```python
from build123d import *

# Parameters (mm, degrees)
CROQUIS1_R              = 5
SALIENTE_EXTRUIR1_DEPTH = 12.5
CROQUIS2_R              = 2
SALIENTE_EXTRUIR2_DEPTH = 10
CROQUIS3_R              = 4
SALIENTE_EXTRUIR3_DEPTH = 15
CROQUIS4_W              = 5.65685425
CROQUIS4_H              = 5.65685425
SALIENTE_EXTRUIR4_DEPTH = 10
CROQUIS5_W              = 4
CROQUIS5_H              = 10
CORTAR_EXTRUIR1_DEPTH   = 2
CROQUIS6_R              = 2.5
SALIENTE_EXTRUIR5_DEPTH = 100


with BuildPart() as part:
    # Croquis1 → Saliente-Extruir1 (new, symmetric)
    with BuildSketch(Plane.XY):
        Circle(CROQUIS1_R)
    extrude(amount=SALIENTE_EXTRUIR1_DEPTH, both=True)

    # Croquis2 → Saliente-Extruir2 (add)
    with BuildSketch(Plane(origin=(0, 0, -12.5), x_dir=(-1, 0, 0), z_dir=(0, 0, -1))):
        Circle(CROQUIS2_R)
    extrude(amount=SALIENTE_EXTRUIR2_DEPTH)

    # Croquis3 → Saliente-Extruir3 (add)
    with BuildSketch(Plane.XY.offset(12.5)):
        Circle(CROQUIS3_R)
    extrude(amount=SALIENTE_EXTRUIR3_DEPTH)

    # Croquis4 → Saliente-Extruir4 (add)
    with BuildSketch(Plane.XY.offset(27.5)):
        Rectangle(CROQUIS4_W, CROQUIS4_H)
    extrude(amount=SALIENTE_EXTRUIR4_DEPTH)

    # Croquis5 → Cortar-Extruir1 (cut)
    with BuildSketch(Plane(origin=(0, 5, 0), x_dir=(1, 0, 0), z_dir=(0, 1, 0))):
        Rectangle(CROQUIS5_W, CROQUIS5_H)
    extrude(amount=-CORTAR_EXTRUIR1_DEPTH, mode=Mode.SUBTRACT)

    # Croquis6 → Saliente-Extruir5 (add)
    with BuildSketch(Plane.XY.offset(37.5)):
        Circle(CROQUIS6_R)
    extrude(amount=SALIENTE_EXTRUIR5_DEPTH)


solid = part.part
```
The listing builds one solid part. Answer for the finished solid, in the listing's coordinates (mm). A direction names the side the tool comes from. Give positions to 0.01 mm unless a question says otherwise; leave off trailing zeros. Order: outer loops, then holes, each group sorted by start corner. A loop starts at its lowest first (then second) coordinate and runs counter-clockwise, first axis right, second up. Notation, with made-up numbers: (13.25, 47) - (20.25, 47) arc R31 cw to (20.25, 79) - close; hole circle Ø7 at (13, -19.75). An arc over 180 degrees is marked (long way). Use one line per item in the form item = value. Start each with the question number.
(1) Flat-ended cylindrical pins translate along their axes: pin 1 Ø2 at (x, z) = (0.5, 1.5) entering from +Y; pin 2 Ø5 at (x, z) = (-2, 120) entering from +Y; pin 3 Ø4 at (x, z) = (-2.5, 98.5) entering from +Y; pin 4 Ø3 at (x, y) = (-3.5, 1.5) entering from +Z. Find the tip coordinate at first contact, or state that the pin passes through.
(2) A cutting plane is placed at D-D, the plane z = 16.5. Write down the section's boundary in (x, y), then the cut area to 3 significant figures.
(3) A cutting plane is placed at A-A, the plane x = 0. Write down the section's boundary in (y, z).
(4) A cutting plane is placed at B-B, the plane y = 0. Write down the section's boundary in (x, z).
(5) The mould has two halves that part along Y. Classify faces 5 (the flat face through (0, -2.828, 32)), 6 (the cylindrical face through (0, -2, -17)), 7 (the flat face through (-2.6, 0.7, 37.5)), 8 (the flat face through (0, 2.828, 32)): released by +Y, released by -Y, zero draft, split by the parting line, or undercut.
(6) A cutting plane is placed at C-C, the plane z = 111.5. Write down the section's boundary in (x, y).
(7) For faces 1 (the flat face through (0, 3, 0)), 2 (the flat face through (-0.1, -2.2, -12.5)), 3 (the flat face through (2.828, 0, 32)), 4 (the cylindrical face through (-0.867, -3.905, 19.895)), determine the directions among +Z, -Z, +X, -X, +Y, -Y from which every point of the face is accessible in a straight line to the end or side of a thin tool.
(8) Consider line 1 (Z direction, x = 0.5, y = 3.5); line 2 (Z direction, x = 1.5, y = -4.5); line 3 (Z direction, x = 0.25, y = -3.5). Determine where each line is inside the solid, lowest interval first. Write a range as from..to.
Ans:
q1.pin_1 = 3
q1.pin_2 = 2.5
q1.pin_3 = 2.45
q1.pin_4 = 137.5
q2.outline = circle Ø8 at (0, 0)
q2.area = 50.3 mm^2
q3.outline = (-5, -12.5) - (-2, -12.5) - (-2, -22.5) - (2, -22.5) - (2, -12.5) - (5, -12.5) - (5, -5) - (3, -5) - (3, 5) - (5, 5) - (5, 12.5) - (4, 12.5) - (4, 27.5) - (2.83, 27.5) - (2.83, 37.5) - (2.5, 37.5) - (2.5, 137.5) - (-2.5, 137.5) - (-2.5, 37.5) - (-2.83, 37.5) - (-2.83, 27.5) - (-4, 27.5) - (-4, 12.5) - (-5, 12.5) - close
q4.outline = (-5, -12.5) - (-2, -12.5) - (-2, -22.5) - (2, -22.5) - (2, -12.5) - (5, -12.5) - (5, 12.5) - (4, 12.5) - (4, 27.5) - (2.83, 27.5) - (2.83, 37.5) - (2.5, 37.5) - (2.5, 137.5) - (-2.5, 137.5) - (-2.5, 37.5) - (-2.83, 37.5) - (-2.83, 27.5) - (-4, 27.5) - (-4, 12.5) - (-5, 12.5) - close
q5.face_5 = released by -Y
q5.face_6 = split by the parting line
q5.face_7 = zero draft
q5.face_8 = released by +Y
q6.outline = circle Ø5 at (0, 0)
q7.face_1 = +Y
q7.face_2 = -Z
q7.face_3 = +Z, +X, +Y, -Y
q7.face_4 = +Z
q8.line_1 = -12.5..-5, 5..27.5
q8.line_2 = -12.5..12.5
q8.line_3 = -12.5..27.5
